from build123d import *

# Parameters (mm, degrees)
SKETCH1_W           = 182.5
SKETCH1_H           = 35
SKETCH1_R           = 4.125
SKETCH1_R_2         = 1.5
BOSS_EXTRUDE1_DEPTH = 3
CUT_EXTRUDE3_START  = 3.5
SKETCH2_W           = 3
SKETCH2_H           = 9.897866997
SKETCH2_W_2         = 27.5
SKETCH2_W_3         = 2
CUT_EXTRUDE3_DEPTH  = 9
SKETCH3_R           = 1.5
CUT_EXTRUDE7_DEPTH  = 10


with BuildPart() as part:
    # Sketch1 → Boss-Extrude1 (new body)
    with BuildSketch(Plane(origin=(0, 0, 0), x_dir=(1, 0, 0), z_dir=(0, 1, 0))):
        with Locations((-8.75, 5)):
            Rectangle(SKETCH1_W, SKETCH1_H)
        with Locations((47.5, 5)):
            Circle(SKETCH1_R, mode=Mode.SUBTRACT)
        with Locations((74.5, 5)):
            Circle(SKETCH1_R_2, mode=Mode.SUBTRACT)
        with Locations((20.5, 5)):
            Circle(SKETCH1_R_2, mode=Mode.SUBTRACT)
        with Locations((-97, -9.5)):
            Circle(SKETCH1_R_2, mode=Mode.SUBTRACT)
        with Locations((-97, -3)):
            Circle(SKETCH1_R_2, mode=Mode.SUBTRACT)
        with Locations((-91.5, 8)):
            Circle(SKETCH1_R_2, mode=Mode.SUBTRACT)
        with Locations((-64, 8)):
            Circle(SKETCH1_R_2, mode=Mode.SUBTRACT)
        with Locations((-64, 1)):
            Circle(SKETCH1_R_2, mode=Mode.SUBTRACT)
        with Locations((-91.5, 1)):
            Circle(SKETCH1_R_2, mode=Mode.SUBTRACT)
    extrude(amount=BOSS_EXTRUDE1_DEPTH)

    # Sketch2 → Cut-Extrude3 (cut)
    with BuildSketch(Plane.XY.offset(CUT_EXTRUDE3_START)):
        with Locations((-90.5, 1.550857661)):
            Rectangle(SKETCH2_W, SKETCH2_H)
        with Locations((-75.25, 1.550857661)):
            Rectangle(SKETCH2_W_2, SKETCH2_H)
        with Locations((-93, 1.550857661)):
            Rectangle(SKETCH2_W_3, SKETCH2_H)
    extrude(amount=CUT_EXTRUDE3_DEPTH, mode=Mode.SUBTRACT)

    # Sketch3 → Cut-Extrude7 (cut)
    with BuildSketch(Plane(origin=(0, 3, 0), x_dir=(-1, 0, 0), z_dir=(0, -1, 0))):
        with Locations((-66.5, -9.307637977)):
            Circle(SKETCH3_R)
        with Locations((-66.5, 19.692362023)):
            Circle(SKETCH3_R)
        with Locations((-28.5, 19.692362023)):
            Circle(SKETCH3_R)
        with Locations((-28.5, -9.307637977)):
            Circle(SKETCH3_R)
    extrude(amount=CUT_EXTRUDE7_DEPTH, mode=Mode.SUBTRACT)


solid = part.part
Source: CAD feature listing. Evaluate the final solid. Frame: model axes, mm. A direction names the side the tool comes from. Round coordinates to 2 decimals unless told otherwise and drop trailing zeros. Loops run counter-clockwise (first coordinate to the right, second up) from the corner with the lowest first, then second, coordinate; pieces in that order, holes last. Notation, with made-up numbers: M 25,26 L 46,26 A20 cw 46,32 Z; hole C 38.25,50.5 d11. An arc over 180 degrees is marked long. Return JSON: item names as keys, results as strings. Group by question number.
1. Section query A-A on x = 28.5. Output: boundary loops of the cut face in (y, z).
2. Mould query, pull axis Z, two halves, no side actions, for faces 3 (the face through (-10, 0, -5)), 4 (the face through (-78, 2, 3.5)), 5 (the face through (-90, 1, -1)), 6 (the face through (-96.194, 1.479, 1.735)). Classes: released by +Z, released by -Z, zero draft, split by the parting line, or undercut.
3. Section query C-C on y = 1.35. State how many separate pieces and enclosed holes the cut face has, and give its area (3 significant figures).
4. Reachability of faces 1 (the face through (-61.5, 1, 8)), 2 (the face through (65.114, 1.521, 9.882)) from +Z, -Z, +X, -X, +Y, -Y: full face, straight path, thin tool, end or side. Return the list, or none.
5. Section query D-D on x = -91.5. Output: boundary loops of the cut face in (y, z).
6. Pin query (flat end, axial travel): pin 1 (1.8 mm diameter, centred on x = 66.5, z = 9.31, fed in from +Y). Return the tip coordinate at first contact, or that it passes through.
7. Material intervals for line 1 along Z through (x, y) = (28.5, 1.05); line 2 along X through (y, z) = (2, -5) (3 decimals); line 3 along Z through (x, y) = (-91.5, 1.8), sorted ascending. Write a range as from..to.
8. Section query B-B on x = 74.5. Output: boundary loops of the cut face in (y, z).
Checks:
{
 "1": {"outline": "M 0,-22.5 L 3,-22.5 L 3,-21.19 L 0,-21.19 Z; M 0,-18.19 L 3,-18.19 L 3,7.81 L 0,7.81 Z; M 0,10.81 L 3,10.81 L 3,12.5 L 0,12.5 Z"},
 "2": {"face 3": "zero draft", "face 4": "released by +Z", "face 5": "undercut", "face 6": "undercut"},
 "3": {"separate pieces": "1", "enclosed holes": "13", "area": "5,960 mm²"},
 "4": {"face 1": "+Z, +Y, -Y", "face 2": "+Y, -Y"},
 "5": {"outline": "M 0,-22.5 L 3,-22.5 L 3,-9.5 L 0,-9.5 Z; M 0,-6.5 L 3,-6.5 L 3,-2.5 L 0,-2.5 Z; M 0,0.5 L 3,0.5 L 3,3.5 L 0,3.5 Z"},
 "6": {"pin 1": "passes through"},
 "7": {"line 1": "z = -22.5..-21.19, -18.19..7.81, 10.81..12.5", "line 2": "x = -100..19, 22..43.375, 51.625..73, 76..82.5", "line 3": "z = -22.5..-9.5, -6.5..-2.5, 0.5..3.5"},
 "8": {"outline": "M 0,-22.5 L 3,-22.5 L 3,-6.5 L 0,-6.5 Z; M 0,-3.5 L 3,-3.5 L 3,12.5 L 0,12.5 Z"}
}
